```python
from build123d import *

# Parameters (mm, degrees)
SKETCH1_W           = 30
SKETCH1_H           = 25
BOSS_EXTRUDE1_DEPTH = 20
CUT_EXTRUDE1_DEPTH  = 50
CUT_EXTRUDE2_DEPTH  = 10


with BuildPart() as part:
    # Sketch1 → Boss-Extrude1 (new body)
    with BuildSketch(Plane.XY):
        with Locations((15, 12.5)):
            Rectangle(SKETCH1_W, SKETCH1_H)
    extrude(amount=BOSS_EXTRUDE1_DEPTH)

    # Sketch2 → Cut-Extrude1 (cut)
    with BuildSketch(Plane.ZY):
        Polygon((15, 25), (20, 15), (20, 25), align=None)
    extrude(amount=-CUT_EXTRUDE1_DEPTH, mode=Mode.SUBTRACT)

    # Sketch3 → Cut-Extrude2 (cut)
    with BuildSketch(Plane(origin=(0, 0, 0), x_dir=(-1, 0, 0), z_dir=(0, 0, -1))):
        Polygon((-20, 25), (-30, 25), (-30, 0), (-25, 0), (-25, 15), align=None)
        Polygon((0, 25), (-10, 25), (-5, 15), (-5, 0), (0, 0), align=None)
    extrude(amount=-CUT_EXTRUDE2_DEPTH, mode=Mode.SUBTRACT)


solid = part.part
```
Check sheet for the modelled part. Datum: model origin and axes. Units: mm. A direction names the side the tool comes from. Coordinates: 2 decimals unless noted, no trailing zeros. Loops run counter-clockwise (first coordinate to the right, second up) from the corner with the lowest first, then second, coordinate; pieces in that order, holes last. Notation, with made-up numbers: M 69,8 L 107,8 A5 ccw 107,16 Z; hole C 72,-7.75 d10. An arc over 180 degrees is marked long. Answer as a JSON object with one key per item and string values.
1. Sectioned sample at C-C on z = 2.25. Record the cut outline in (x, y), and give its area (3 significant figures).
Outcome:
{"outline": "M 5,0 L 25,0 L 25,15 L 20,25 L 10,25 L 5,15 Z", "area": "450 mm²"}
2. Sectioned sample at B-B on x = 9.5. Record the cut outline in (y, z), and give its area (3 significant figures).
Outcome:
{"outline": "M 0,0 L 24,0 L 24,10 L 25,10 L 25,15 L 15,20 L 0,20 Z", "area": "465 mm²"}
3. Depth check by flat-ended pin: P1, Ø4, axis at y = 15.5, z = 6, coming from the -X side. Enter the tip coordinate at first touch or a pass-through.
Outcome:
{"P1": "x = 5"}
4. Sectioned sample at D-D on y = 17.5. Record the cut outline in (x, z), and give its area (4 significant figures).
Outcome:
{"outline": "M 0,10 L 6.25,10 L 6.25,0 L 23.75,0 L 23.75,10 L 30,10 L 30,18.75 L 0,18.75 Z", "area": "437.5 mm²"}
5. Scan lines: L1, parallel to Z at x = 25.5, y = 12; L2, parallel to X at y = 2.25, z = 6.25; L3, parallel to Y at x = 22.5, z = 18.75. Record each from-to range of solid material in increasing order. Write a range as from..to.
Outcome:
{"L1": "10..20", "L2": "5..25", "L3": "0..17.5"}
6. Sectioned sample at A-A on y = 13.25. Record the cut outline in (x, z), and give its area (3 significant figures).
Outcome:
{"outline": "M 0,10 L 5,10 L 5,0 L 25,0 L 25,10 L 30,10 L 30,20 L 0,20 Z", "area": "500 mm²"}
7. Access from +Z, -Z, +X, -X, +Y, -Y to the whole of each face (thin tool, end or side, straight path). Record for faces 1 (the flat face through (5, 8, 5)), 2 (the flat face through (7.535, 20.07, 4.93)), 3 (the flat face through (22.535, 19.93, 4.93)).
Outcome:
{"face 1": "-Z, -X, +Y, -Y", "face 2": "-Z, -X, +Y", "face 3": "-Z, +X, +Y"}
